Autodesk Inventor part; units mm, degrees
ref_plane "Work Plane2" through (-34.82, -48.575, 205.34) normal (0, 0, -1) x (0, 1, 0)
ref_plane "YZ Plane" through (0, 0, 0) normal (1, 0, 0) x (0, 1, 0)
ref_plane "XZ Plane" through (0, 0, 0) normal (0, 1, 0) x (-1, 0, 0)
ref_plane "Work Plane1" through (0, 0, 0) normal (0, 0, 1) x (1, 0, 0)
sketch "Sketch1" plane through (0, 0, 0) normal (0, 0, 1) x (1, 0, 0)
  circle A0 centre (-23.32, -39.075) radius 2.355
  circle A1 centre (-23.32, 39.075) radius 2.355
  circle A2 centre (20.82, -6.975) radius 2
  circle A3 centre (20.82, 7.075) radius 2
  line L0 (32.82, 48.575) -> (-32.82, 48.575)
  arc A4 (-32.82, 48.575) -> (-34.82, 46.575) centre (-32.82, 46.575) ccw
  line L1 (-34.82, 46.575) -> (-34.82, -46.575)
  arc A5 (-34.82, -46.575) -> (-32.82, -48.575) centre (-32.82, -46.575) ccw
  line L2 (-32.82, -48.575) -> (32.82, -48.575)
  arc A6 (32.82, -48.575) -> (34.82, -46.575) centre (32.82, -46.575) ccw
  line L3 (34.82, -46.575) -> (34.82, 46.575)
  arc A7 (34.82, 46.575) -> (32.82, 48.575) centre (32.82, 46.575) ccw
  line L4 (13.32, -15) -> (28.32, 15) construction
  line L5 (28.32, -15) -> (13.32, 15) construction
  line L6 (32.32, 10.075) -> (24.32, 10.075)
  line L7 (24.32, 10.075) -> (24.32, 4.075)
  line L8 (24.32, 4.075) -> (32.32, 4.075)
  line L9 (32.32, 4.075) -> (32.32, 10.075)
  line L10 (32.32, 10.075) -> (24.32, 4.075) construction
  line L11 (24.32, 10.075) -> (32.32, 4.075) construction
  line L12 (32.32, -3.975) -> (24.32, -3.975)
  line L13 (24.32, -3.975) -> (24.32, -9.975)
  line L14 (24.32, -9.975) -> (32.32, -9.975)
  line L15 (32.32, -9.975) -> (32.32, -3.975)
  line L16 (32.32, -3.975) -> (24.32, -9.975) construction
  line L17 (24.32, -3.975) -> (32.32, -9.975) construction
  line L18 (9.32, 4.075) -> (17.32, 4.075)
  line L19 (17.32, 4.075) -> (17.32, 10.075)
  line L20 (17.32, 10.075) -> (9.32, 10.075)
  line L21 (9.32, 10.075) -> (9.32, 4.075)
  line L22 (9.32, 4.075) -> (17.32, 10.075) construction
  line L23 (17.32, 4.075) -> (9.32, 10.075) construction
  line L24 (9.32, -9.975) -> (17.32, -9.975)
  line L25 (17.32, -9.975) -> (17.32, -3.975)
  line L26 (17.32, -3.975) -> (9.32, -3.975)
  line L27 (9.32, -3.975) -> (9.32, -9.975)
  line L28 (9.32, -9.975) -> (17.32, -3.975) construction
  line L29 (17.32, -9.975) -> (9.32, -3.975) construction
  line L30 (23.82, 19) -> (17.82, 19)
  line L31 (17.82, 19) -> (17.82, 11)
  line L32 (17.82, 11) -> (23.82, 11)
  line L33 (23.82, 11) -> (23.82, 19)
  line L34 (23.82, 19) -> (17.82, 11) construction
  line L35 (17.82, 19) -> (23.82, 11) construction
  line L36 (17.82, -19) -> (23.82, -19)
  line L37 (23.82, -19) -> (23.82, -11)
  line L38 (23.82, -11) -> (17.82, -11)
  line L39 (17.82, -11) -> (17.82, -19)
  line L40 (17.82, -19) -> (23.82, -11) construction
  line L41 (23.82, -19) -> (17.82, -11) construction
  line L42 (28.32, 15) -> (23.82, 15)
  line L43 (17.82, 15) -> (13.32, 15)
  line L44 (28.32, 10.075) -> (28.32, 15)
  line L45 (28.32, -15) -> (28.32, -9.975)
  line L46 (28.32, -3.975) -> (28.32, 4.075)
  line L47 (13.32, -15) -> (17.82, -15)
  line L48 (23.82, -15) -> (28.32, -15)
  line L49 (13.32, -9.975) -> (13.32, -15)
  line L50 (13.32, 15) -> (13.32, 10.075)
  line L51 (13.32, 4.075) -> (13.32, -3.975)
  point P0 (0, 0)
  point P1 (20.82, 0)
  dimension "d0" = 15
  dimension "d1" = 30
  dimension "d2" = 8
  dimension "d3" = 6
  dimension "d4" = 6
  dimension "d5" = 8
  dimension "d6" = 6
  dimension "d7" = 8
  dimension "d8" = 6
  dimension "d9" = 8
ref_plane "Work Plane2" through (-34.82, -48.575, 205.34) normal (0, 0, -1) x (0, 1, 0)
extrude "Extrusion1" add sketch "Sketch1" along normal up to surface (205.34 mm away) contours L6 L7 L8 L46 L12 L13 L14 L45 L48 L37 L38 L39 L47 L49 L24 L25 L26 L51 L18 L19 L20 L50 L43 L31 L32 L33 L42 L44
properties part number "Neje_Aluminium_Slide_X"
Model file for the job. Use its own axes, mm. A direction names the side the tool comes from. Give positions to 0.01 mm unless a question says otherwise; leave off trailing zeros. Loops run counter-clockwise (first coordinate to the right, second up) from the corner with the lowest first, then second, coordinate; pieces in that order, holes last.
Item 1: Slice it at C-C (z = 168.5). Give the number of separate pieces and of enclosed holes in the cut face, plus the area to 3 significant figures.
Check values:
separate pieces: 1
enclosed holes: 2
area: 281 mm2
Item 2: Slice it at B-B (y = 13). Write the cut outline in (x, z).
Check values:
outline: (13.32, 0) - (17.82, 0) - (17.82, 205.34) - (13.32, 205.34) - close; (23.82, 0) - (28.32, 0) - (28.32, 205.34) - (23.82, 205.34) - close
Item 3: Drop flat-ended pins along their axis: P1, Ø3, axis at y = -7, z = 129, coming from the -X side; P2, Ø5, axis at x = 20.5, z = 89, coming from the +Y side. Give the stop position or say it passes through.
Check values:
P1: stops at x = 17.32
P2: stops at y = 11
Item 4: Drill centre lines: line 1 along Y through (x, z) = (20.82, 56) (3 decimals); line 2 along Y through (x, z) = (15, 114) (3 decimals); line 3 along X through (y, z) = (13.75, 43.5). Where is each one in solid material? Low to high.
Check values:
line 1: y = -11 to -8.975, -4.975 to 5.075, 9.075 to 11
line 2: y = -15 to -9.975, -3.975 to 4.075, 10.075 to 15
line 3: x = 13.32 to 17.82, 23.82 to 28.32
Item 5: Mould opens along Y. For faces 1 (the face through (17.32, -7, 101)), 2 (the face through (16, 15, 101)), 3 (the face through (13.32, 0, 101)) say: +Y half, -Y half, draft (parallel to the pull), parting line (faces both ways), or undercut.
Check values:
face 1: undercut
face 2: +Y half
face 3: draft
Item 6: Slice it at A-A (x = 15). Write the cut outline in (y, z) (3 decimals), plus the area to 3 significant figures.
Check values:
outline: (-15, 0) - (-9.975, 0) - (-9.975, 205.34) - (-15, 205.34) - close; (-3.975, 0) - (4.075, 0) - (4.075, 205.34) - (-3.975, 205.34) - close; (10.075, 0) - (15, 0) - (15, 205.34) - (10.075, 205.34) - close
area: 3,700 mm2
Item 7: Which spindle directions (+Z, -Z, +X, -X, +Y, -Y) get a long thin tool onto all of the face, cutting with end or side? Do faces 4 (the face through (26, -3.975, 101)), 5 (the face through (23.82, 13, 101)), 6 (the face through (17.32, 7, 101)), 7 (the face through (23.82, -13, 101)). Say none if no direction does.
Check values:
face 4: +Z, -Z, +X
face 5: +Z, -Z, +Y
face 6: +Z, -Z, -X
face 7: +Z, -Z, -Y
